Can you work these out from the model? Positions are in its coordinate system, mm. Face numbers are marked on the shaded views. A direction names the side the tool comes from. Give positions to 0.01 mm unless a question says otherwise; leave off trailing zeros. Write each loop counter-clockwise with the first axis right and the second up, starting at its lowest first coordinate (ties: lowest second). Pieces come first, ordered by that corner, then holes.
```python
from build123d import *

# Parameters (mm, degrees)
SKETCH1_W           = 80
SKETCH1_H           = 175
SKETCH1_R           = 2.5
BOSS_EXTRUDE1_DEPTH = 1
SKETCH2_W           = 175
SKETCH2_H           = 150
BOSS_EXTRUDE2_DEPTH = 1
SKETCH3_W           = 60
SKETCH3_H           = 175
BOSS_EXTRUDE3_DEPTH = 1


with BuildPart() as part:
    # Sketch1 → Boss-Extrude1 (new body)
    with BuildSketch(Plane(origin=(0, 0, 0), x_dir=(1, 0, 0), z_dir=(0, 1, 0))):
        Rectangle(SKETCH1_W, SKETCH1_H)
        with Locations(Location((-4, 19.6, 0), (0, 0, 270))):
            Circle(SKETCH1_R, mode=Mode.SUBTRACT)
        with Locations(Location((-4, -19.6, 0), (0, 0, 90))):
            Circle(SKETCH1_R, mode=Mode.SUBTRACT)
    extrude(amount=BOSS_EXTRUDE1_DEPTH)

    # Sketch2 → Boss-Extrude2 (add)
    with BuildSketch(Plane(origin=(40, 0, 0), x_dir=(0, 0, -1), z_dir=(1, 0, 0))):
        with Locations((0, 75)):
            Rectangle(SKETCH2_W, SKETCH2_H)
    extrude(amount=BOSS_EXTRUDE2_DEPTH)

    # Sketch3 → Boss-Extrude3 (add)
    with BuildSketch(Plane(origin=(0, 150, 0), x_dir=(1, 0, 0), z_dir=(0, 1, 0))):
        with Locations((70, 0)):
            Rectangle(SKETCH3_W, SKETCH3_H)
    extrude(amount=BOSS_EXTRUDE3_DEPTH)


solid = part.part
```
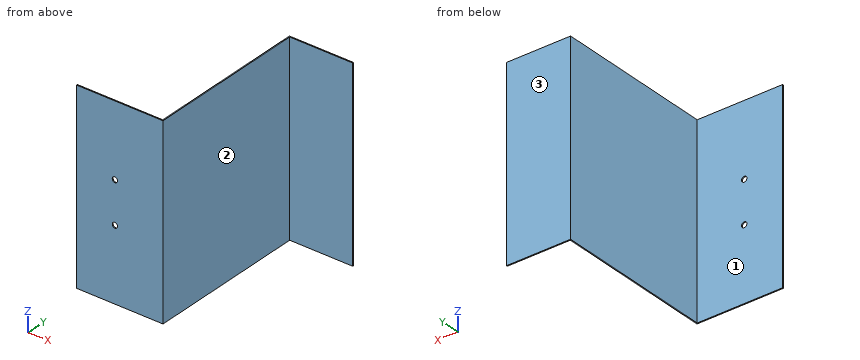
1) Suppose I cut it at B-B on z = 19.6. Write out the boundary of the cut face in (x, y), plus the area to 3 significant figures.
Values follow:
outline: (-40, 0) - (-6.5, 0) - (-6.5, 1) - (-40, 1) - close; (-1.5, 0) - (41, 0) - (41, 150) - (100, 150) - (100, 151) - (40, 151) - (40, 1) - (-1.5, 1) - close
area: 285 mm2
2) Suppose I cut it at A-A on x = -4. Write out the boundary of the cut face in (y, z).
Values follow:
outline: (0, -87.5) - (1, -87.5) - (1, -22.1) - (0, -22.1) - close; (0, -17.1) - (1, -17.1) - (1, 17.1) - (0, 17.1) - close; (0, 22.1) - (1, 22.1) - (1, 87.5) - (0, 87.5) - close
3) For the marked faces 1, 2 and 3, which set-ups out of +Z, -Z, +X, -X, +Y, -Y let a thin tool reach every point of the face, with its end or its side?
Values follow:
face 1: +Z, -Z, -X, +Y
face 2: +Z, -Z, +X, -Y
face 3: +Z, -Z, +X, -X, +Y
4) Suppose I cut it at C-C on y = 113. Write out the boundary of the cut face in (x, z), plus the area to 3 significant figures.
Values follow:
outline: (40, -87.5) - (41, -87.5) - (41, 87.5) - (40, 87.5) - close
area: 175 mm2
5) For pin 1 Ø1 at (x, z) = (-7.5, -5.5) entering from +Y; pin 2 Ø3 at (x, z) = (-4, 19.6) entering from +Y; pin 3 Ø3 at (x, z) = (82.5, -3.5) entering from -Y, each with a flat end and sliding along its axis, tell me the tip position at first contact or that it passes through.
Values follow:
pin 1: stops at y = 1
pin 2: passes through
pin 3: stops at y = 150
6) Suppose I cut it at D-D on z = 41. Write out the boundary of the cut face in (x, y).
Values follow:
outline: (-40, 0) - (41, 0) - (41, 150) - (100, 150) - (100, 151) - (40, 151) - (40, 1) - (-40, 1) - close
7) Please list where these lines run through material, in increasing order: L1, parallel to Y at x = -27, z = 72.5; L2, parallel to X at y = 0.65, z = -19.6; L3, parallel to X at y = 58.5, z = 17.
Values follow:
L1: y = 0 to 1
L2: x = -40 to -6.5, -1.5 to 41
L3: x = 40 to 41
